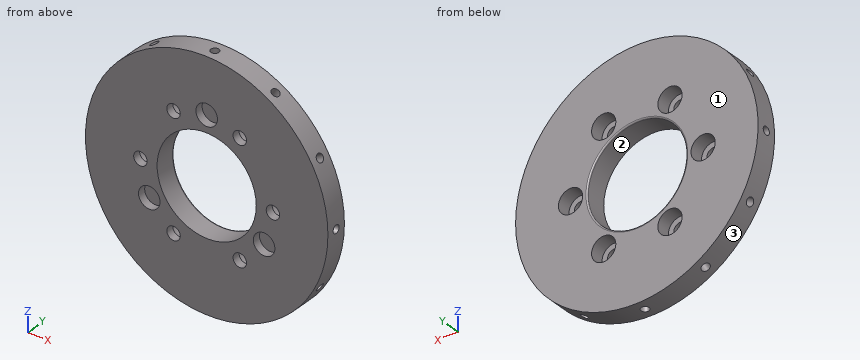
from build123d import *

# Parameters (mm, degrees)
SKETCH_1_R               = 45
SKETCH_1_R_2             = 2.5
SKETCH_1_R_3             = 18.4
EXTRUDE_1_DEPTH          = 8
SKETCH_2_R               = 4
CUT_EXTRUDE_1_DEPTH      = 3
SKETCH_4_R               = 4.5
CUT_EXTRUDE_2_DEPTH      = 5.1
SKETCH_5_R               = 1.5
CUT_EXTRUDE_3_DEPTH      = 10
PATTERN_CIRCULAR_1_COUNT = 12
FILLET_1_R               = 0.5


with BuildPart() as part:
    # 草图1 → 凸台-拉伸1 (new body)
    with BuildSketch(Plane(origin=(0, 0, 0), x_dir=(1, 0, 0), z_dir=(0, 1, 0))):
        Circle(SKETCH_1_R)
        with Locations((-24.6, 0)):
            Circle(SKETCH_1_R_2, mode=Mode.SUBTRACT)
        with Locations((-12.3, 21.304224933)):
            Circle(SKETCH_1_R_2, mode=Mode.SUBTRACT)
        with Locations((12.3, 21.304224933)):
            Circle(SKETCH_1_R_2, mode=Mode.SUBTRACT)
        with Locations((24.6, 0)):
            Circle(SKETCH_1_R_2, mode=Mode.SUBTRACT)
        with Locations((12.3, -21.304224933)):
            Circle(SKETCH_1_R_2, mode=Mode.SUBTRACT)
        with Locations((-12.3, -21.304224933)):
            Circle(SKETCH_1_R_2, mode=Mode.SUBTRACT)
        Circle(SKETCH_1_R_3, mode=Mode.SUBTRACT)
    extrude(amount=EXTRUDE_1_DEPTH)

    # 草图2 → 切除-拉伸1 (cut)
    with BuildSketch(Plane.XZ):
        with Locations((-21.304224933, -12.3)):
            Circle(SKETCH_2_R)
        with Locations((0, 24.6)):
            Circle(SKETCH_2_R)
        with Locations((21.304224933, -12.3)):
            Circle(SKETCH_2_R)
    extrude(amount=-CUT_EXTRUDE_1_DEPTH, mode=Mode.SUBTRACT)

    # 草图4 → 切除-拉伸2 (cut)
    with BuildSketch(Plane(origin=(0, 8, 0), x_dir=(1, 0, 0), z_dir=(0, 1, 0))):
        with Locations((-24.6, 0)):
            Circle(SKETCH_4_R)
        with Locations((-12.3, 21.304224933)):
            Circle(SKETCH_4_R)
        with Locations((12.3, 21.304224933)):
            Circle(SKETCH_4_R)
        with Locations((24.6, 0)):
            Circle(SKETCH_4_R)
        with Locations((12.3, -21.304224933)):
            Circle(SKETCH_4_R)
        with Locations((-12.3, -21.304224933)):
            Circle(SKETCH_4_R)
    extrude(amount=-CUT_EXTRUDE_2_DEPTH, mode=Mode.SUBTRACT)

    # 草图5 → 切除-拉伸3 (cut)
    with BuildSketch(Plane(origin=(45, 0, 0), x_dir=(0, 0, -1), z_dir=(1, 0, 0))):
        with Locations((0, 4)):
            Circle(SKETCH_5_R)
    cut_extrude_3 = extrude(amount=-CUT_EXTRUDE_3_DEPTH, mode=Mode.SUBTRACT)

    # 阵列(圆周)1: 切除-拉伸3 ×12 about axis
    pattern_circular_1_axis = Axis((0, 0, 0), (0, 1, 0))
    for i in range(1, PATTERN_CIRCULAR_1_COUNT):
        add(cut_extrude_3.rotate(pattern_circular_1_axis, i * 360 / PATTERN_CIRCULAR_1_COUNT), mode=Mode.SUBTRACT)

    # 圆角1
    fillet_1_edges = [part.edges().sort_by_distance(p)[0] for p in [
        (-18.4, 8, 0),
    ]]
    fillet(fillet_1_edges, radius=FILLET_1_R)


solid = part.part
Work out the finished part from the listing and answer in its coordinate system (mm). Face numbers are marked on the shaded views. Coordinates: 2 decimals unless noted, no trailing zeros. Write each question's results on one line, items separated by ' | '. Start each with the question number.
1) The mould has two halves that part along Z. Classify the marked faces 1, 2 and 3: pulls with the +Z half, pulls with the -Z half, needs draft (parallel to the pull), parting line crosses it, or undercut.
2) Find section A-A on z = 0. Count the separate pieces of the cut face and the enclosed holes in it, then the cut area to 3 significant figures.
3) Flat-ended cylindrical pins translate along their axes: P1, Ø2.5, axis at x = -21.5, z = -12, coming from the -Y side; P2, Ø6.5, axis at x = -24.6, z = 0, coming from the +Y side; P3, Ø3, axis at y = 6, z = 27.5, coming from the -X side; P4, Ø3, axis at x = 12.3, z = -21.3, coming from the -Y side. Find the tip coordinate at first contact, or state that the pin passes through.
4) Consider line 1 along X through (y, z) = (1.05, 0); line 2 along X through (y, z) = (5.35, 0); line 3 along Y through (x, z) = (31, 18). Determine where each line is inside the solid, lowest interval first.
Response values:
1) face 1: needs draft | face 2: undercut | face 3: parting line crosses it
2) separate pieces: 4 | enclosed holes: 0 | area: 245 mm^2
3) P1: stops at y = 3 | P2: stops at y = 2.9 | P3: stops at x = -36.73 | P4: passes through
4) line 1: x = -45 to -27.1, -22.1 to -18.4, 18.4 to 22.1, 27.1 to 45 | line 2: x = -35 to -29.1, -20.1 to -18.4, 18.4 to 20.1, 29.1 to 35 | line 3: y = 0 to 2.5, 5.5 to 8
